```python
from build123d import *

# Parameters (mm, degrees)
SKETCH1_R           = 6.35
BOSS_EXTRUDE1_DEPTH = 12.7
CUT_EXTRUDE1_DEPTH  = 9.525
SKETCH3_W           = 5.08
SKETCH3_H           = 5.08
CUT_EXTRUDE2_DEPTH  = 9.525
CHAMFER1_SIZE       = 0.508


with BuildPart() as part:
    # Sketch1 → Boss-Extrude1 (new body)
    with BuildSketch(Plane.XY):
        Circle(SKETCH1_R)
    extrude(amount=BOSS_EXTRUDE1_DEPTH)

    # Sketch2 → Cut-Extrude1 (cut)
    with BuildSketch(Plane.XY.offset(12.7)):
        Polygon((0, -5.499261314), (4.7625, -2.749630657), (4.7625, 2.749630657), (0, 5.499261314), (-4.7625, 2.749630657), (-4.7625, -2.749630657), align=None)
    extrude(amount=-CUT_EXTRUDE1_DEPTH, mode=Mode.SUBTRACT)

    # Sketch3 → Cut-Extrude2 (cut)
    with BuildSketch(Plane.XY.offset(3.175)):
        Rectangle(SKETCH3_W, SKETCH3_H)
    extrude(amount=-CUT_EXTRUDE2_DEPTH, mode=Mode.SUBTRACT)

    # Chamfer1
    chamfer1_edges = [part.edges().sort_by_distance(p)[0] for p in [
        (-6.35, 0, 12.7),
    ]]
    chamfer(chamfer1_edges, length=CHAMFER1_SIZE)


solid = part.part
```
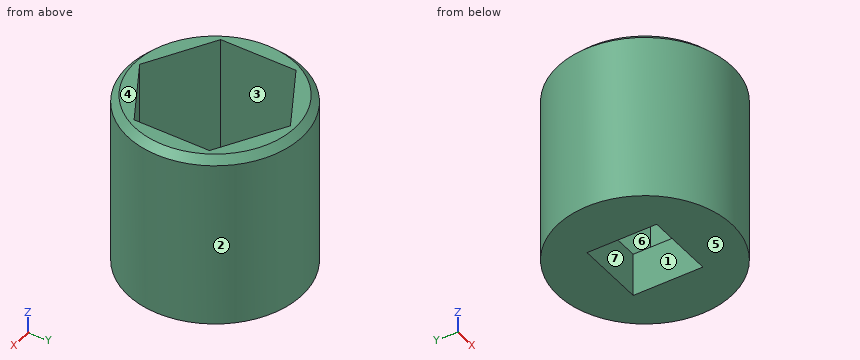
Could you check a few things on this model? Use its own coordinates, in mm. Face numbers are marked on the shaded views. A direction names the side the tool comes from. Give positions to 0.01 mm unless a question says otherwise; leave off trailing zeros. Loops run counter-clockwise (first coordinate to the right, second up) from the corner with the lowest first, then second, coordinate; pieces in that order, holes last. Notation, with made-up numbers: (6.5, 2) - (30.5, 2) arc R14 cw to (30.5, 19) - close; hole circle Ø5 at (-24, -36.75). An arc over 180 degrees is marked (long way). Answer in a Markdown table with one row per item. Add a question column.
Q1. Please list where these lines run through material, in increasing order: L1, parallel to Z at x = -1.25, y = -3 (3 decimals); L2, parallel to X at y = 2, z = 8; L3, parallel to X at y = -5, z = 11.5. Write a range as from..to.
Q2. We'd pull the mould along Y, two halves only. Please class the marked faces 1, 2, 3 and 4: +Y half, -Y half, draft (parallel to the pull), parting line (faces both ways), or undercut.
Q3. If we section it at B-B (z = 5): List the corners of the cut face in (x, y) for me, plus the area to 3 significant figures.
Q4. For pin 1 (1 mm diameter, centred on y = -2, z = 10.5, fed in from -X); pin 2 (1.5 mm diameter, centred on x = 4, z = 5.5, fed in from +Y); pin 3 (1.5 mm diameter, centred on x = 2.5, z = 3.5, fed in from -Y), each with a flat end and sliding along its axis, tell me the tip position at first contact or that it passes through.
Q5. Which directions (+Z, -Z, +X, -X, +Y, -Y) give clear straight access to the entire face, cutting with the end or side of a thin tool? Please do the marked faces 5, 6 and 7.
The answers:
| question | item | result |
|---|---|---|
| 1 | L1 | z = 0..3.175 |
| 1 | L2 | x = -6.03..-4.76, 4.76..6.03 |
| 1 | L3 | x = -3.91..-0.86, 0.86..3.91 |
| 2 | face 1 | undercut |
| 2 | face 2 | parting line |
| 2 | face 3 | undercut |
| 2 | face 4 | draft |
| 3 | outline | circle Ø12.7 at (0, 0); hole (-4.76, -2.75) - (0, -5.5) - (4.76, -2.75) - (4.76, 2.75) - (0, 5.5) - (-4.76, 2.75) - close |
| 3 | area | 48.1 mm^2 |
| 4 | pin 1 | stops at x = -6.17 |
| 4 | pin 2 | stops at y = 5.46 |
| 4 | pin 3 | stops at y = -6.1 |
| 5 | face 5 | -Z, +X, -X, +Y, -Y |
| 5 | face 6 | +Z |
| 5 | face 7 | +Z, -Z |
